```python
from build123d import *

# Parameters (mm, degrees)
F1_DEPTH = 38.1
F3_DEPTH = 25.4
F4_R     = 6.35
F5_DEPTH = 12.701
F6_R     = 3.175
F7_DEPTH = 6.351


with BuildPart() as f1:
    # F0 (on Front) → F1 (new body)
    with BuildSketch(Plane.XZ):
        with BuildLine():
            ThreePointArc((-42.129658, 53.987246), (-51.109914, 50.267503), (-54.829658, 41.287246))
            Line((-54.829658, 41.287246), (-54.829658, 9.537246))
            Line((-54.829658, 9.537246), (8.670342, 9.537246))
            Line((8.670342, 9.537246), (8.670342, 15.887246))
            Line((8.670342, 15.887246), (-16.729658, 15.887246))
            ThreePointArc((-16.729658, 15.887246), (-26.059538, 27.117037), (-29.429707, 41.322558))
            ThreePointArc((-29.429707, 41.322558), (-33.161895, 50.279978), (-42.129658, 53.987246))
        make_face()
    extrude(amount=F1_DEPTH)

    # F2 (on face) → F3 (cut)
    with BuildSketch(Plane.XZ.offset(38.1)):
        with BuildLine():
            Line((-54.829658, 15.887246), (-16.729658, 15.887246))
            ThreePointArc((-16.729658, 15.887246), (-26.059538, 27.117037), (-29.429707, 41.322558))
            ThreePointArc((-29.429707, 41.322558), (-42.147313, 53.987234), (-54.829658, 41.287246))
            Line((-54.829658, 41.287246), (-54.829658, 15.887246))
        make_face()
    extrude(amount=-F3_DEPTH, mode=Mode.SUBTRACT)

    # F4 (on face) → F5 (cut, through all)
    with BuildSketch(Plane.XZ.offset(12.7)):
        with Locations((-42.129658, 41.287246)):
            Circle(F4_R)
    extrude(amount=-F5_DEPTH, mode=Mode.SUBTRACT)

    # F6 (on face) → F7 (cut, through all)
    with BuildSketch(Plane.XY.offset(15.887246)):
        with Locations((-0.854658, -6.692464)):
            Circle(F6_R)
        with Locations((-0.854658, -28.575)):
            Circle(F6_R)
        with Locations((-45.304658, -28.575)):
            Circle(F6_R)
    extrude(amount=-F7_DEPTH, mode=Mode.SUBTRACT)


solid = f1.part
```
Geometry check sheet. Reference: the model listing, model coordinates, mm. A direction names the side the tool comes from. Round coordinates to 2 decimals unless told otherwise and drop trailing zeros. Loops run counter-clockwise (first coordinate to the right, second up) from the corner with the lowest first, then second, coordinate; pieces in that order, holes last. Notation, with made-up numbers: (61.5, 45.25) -> (111.5, 45.25) arc R14 cw to (111.5, 51.25) -> close; hole circle Ø8 at (69.25, 63.25). An arc over 180 degrees is marked (long way). Use a Markdown table: item, result.
(1) Sectioned sample at A-A (y = -9). Enter the section's corners in (x, z).
Calculated:
| item | result |
|---|---|
| outline | (-54.83, 9.54) -> (-3.04, 9.54) -> (-3.04, 15.89) -> (-16.73, 15.89) arc R32 cw to (-29.43, 41.32) arc R12.7 ccw to (-42.13, 53.99) arc R12.7 ccw to (-54.83, 41.29) -> close; (1.33, 9.54) -> (8.67, 9.54) -> (8.67, 15.89) -> (1.33, 15.89) -> close; hole circle Ø12.7 at (-42.13, 41.29) |
(2) Sectioned sample at C-C (z = 37.5). Enter the section's corners in (x, y), then the cut area to 3 significant figures.
Calculated:
| item | result |
|---|---|
| outline | (-54.83, -12.7) -> (-47.23, -12.7) -> (-47.23, 0) -> (-54.83, 0) -> close; (-37.03, -12.7) -> (-29.19, -12.7) -> (-29.19, 0) -> (-37.03, 0) -> close |
| area | 196 mm² |
(3) Set-up check for faces 4 (the flat face through (-40, -12.7, 31)), 5 (the cylindrical face through (-1.5, -9.8, 12.8)): record each of +Z, -Z, +X, -X, +Y, -Y from which the full face is reachable in a straight line by a thin tool's end or side.
Calculated:
| item | result |
|---|---|
| face 4 | +Z, +X, -X, -Y |
| face 5 | +Z, -Z |
(4) Mould release check, pull along Y, two halves, no side actions. Record for faces 1 (the flat face through (-23, -23, 15.887)), 2 (the cylindrical face through (-42.276, -27.621, 12.757)), 3 (the flat face through (-38, 0, 27)): released by +Y, released by -Y, zero draft, split by the parting line, or undercut.
Calculated:
| item | result |
|---|---|
| face 1 | zero draft |
| face 2 | undercut |
| face 3 | released by +Y |
(5) Go/stop test with flat-tipped pins: P1, Ø7.5, axis at x = -42.13, z = 41.29, coming from the -Y side (1 decimal); P2, Ø6, axis at x = -29.5, z = 31, coming from the +Y side; P3, Ø12, axis at x = -33.5, z = 28, coming from the -Y side; P4, Ø4, axis at x = -35.5, y = -8.5, coming from the +Z side. Record where each tip stops, or that it passes through.
Calculated:
| item | result |
|---|---|
| P1 | through |
| P2 | y = 0 |
| P3 | y = -12.7 |
| P4 | z = 53.11 |
(6) Sectioned sample at B-B (x = -1). Enter the section's corners in (y, z), then the cut area to 3 significant figures.
Calculated:
| item | result |
|---|---|
| outline | (-38.1, 9.54) -> (-31.75, 9.54) -> (-31.75, 15.89) -> (-38.1, 15.89) -> close; (-25.4, 9.54) -> (-9.86, 9.54) -> (-9.86, 15.89) -> (-25.4, 15.89) -> close; (-3.52, 9.54) -> (0, 9.54) -> (0, 15.89) -> (-3.52, 15.89) -> close |
| area | 161 mm² |
(7) Scan lines: probe 1 along Y at (x, z) = (-33.5, 33.5); probe 2 along Z at (x, y) = (-43.5, -34.5); probe 3 along X at (y, z) = (-26, 15). Record each from-to range of solid material in increasing order.
Calculated:
| item | result |
|---|---|
| probe 1 | -12.7 to 0 |
| probe 2 | 9.54 to 15.89 |
| probe 3 | -54.83 to -47.16, -43.45 to -2.71, 1 to 8.67 |
(8) Sectioned sample at D-D (y = -31). Enter the section's corners in (x, z).
Calculated:
| item | result |
|---|---|
| outline | (-54.83, 9.54) -> (-47.35, 9.54) -> (-47.35, 15.89) -> (-54.83, 15.89) -> close; (-43.26, 9.54) -> (-2.9, 9.54) -> (-2.9, 15.89) -> (-43.26, 15.89) -> close; (1.19, 9.54) -> (8.67, 9.54) -> (8.67, 15.89) -> (1.19, 15.89) -> close |
